```python
from build123d import *

# Parameters (mm, degrees)
F0_W     = 50.8
F0_H     = 50.8
F1_DEPTH = 50.8
F2_W     = 25.4
F2_H     = 25.4
F3_DEPTH = 25.4
F4_W     = 25.4
F4_H     = 25.4
F5_DEPTH = 25.4
F6_R     = 12.703868
F7_DEPTH = 25.4
F8_R     = 14.195008
F9_DEPTH = 25.4


with BuildPart() as f1:
    # F0 (on Front) → F1 (new body)
    with BuildSketch(Plane.XZ):
        with Locations((-25.4, 25.4)):
            Rectangle(F0_W, F0_H)
    extrude(amount=F1_DEPTH)

    # F2 (on face) → F3 (join)
    with BuildSketch(Plane.XZ.offset(50.8)):
        with Locations((-25.4, 25.4)):
            Rectangle(F2_W, F2_H)
    extrude(amount=F3_DEPTH)

    # F4 (on face) → F5 (cut)
    with BuildSketch(Plane(origin=(-50.8, 0, 0), x_dir=(0, -1, 0), z_dir=(-1, 0, 0))):
        with Locations((25.4, 25.4)):
            Rectangle(F4_W, F4_H)
    extrude(amount=-F5_DEPTH, mode=Mode.SUBTRACT)

    # F6 (on face) → F7 (cut)
    with BuildSketch(Plane.YZ):
        with Locations((-25.396969, 23.869332)):
            Circle(F6_R)
    extrude(amount=-F7_DEPTH, mode=Mode.SUBTRACT)

    # F8 (on face) → F9 (join)
    with BuildSketch(Plane(origin=(0, 0, 0), x_dir=(-1, 0, 0), z_dir=(0, 1, 0))):
        with Locations((24.574604, 25.969833)):
            Circle(F8_R)
    extrude(amount=F9_DEPTH)


solid = f1.part
```
Work out the finished part from the listing and answer in its coordinate system (mm). A direction names the side the tool comes from. Round coordinates to 2 decimals unless told otherwise and drop trailing zeros. Loops run counter-clockwise (first coordinate to the right, second up) from the corner with the lowest first, then second, coordinate; pieces in that order, holes last.
(1) Each of these flat-tipped pins is pushed along its axis until it touches: P1, Ø3.5, axis at y = -17, z = 16, coming from the -X side; P2, Ø15.5, axis at y = -27, z = 30.5, coming from the -X side; P3, Ø7.5, axis at x = -31, y = -69.5, coming from the +Z side; P4, Ø20.5, axis at x = -20.5, y = -64.5, coming from the -Z side. Where does it stop, or does it pass through?
Computed values:
P1: stops at x = -25.4
P2: stops at x = -50.8
P3: stops at z = 38.1
P4: stops at z = 12.7
(2) The part is cut by section C-C, the plane x = -36. Give the vertices of the cut face in (y, z), and give its area (3 significant figures).
Computed values:
outline: (-76.2, 12.7) - (-50.8, 12.7) - (-50.8, 0) - (0, 0) - (0, 17.55) - (25.4, 17.55) - (25.4, 34.39) - (0, 34.39) - (0, 50.8) - (-50.8, 50.8) - (-50.8, 38.1) - (-76.2, 38.1) - close; hole (-38.1, 12.7) - (-12.7, 12.7) - (-12.7, 38.1) - (-38.1, 38.1) - close
area: 3,010 mm2
(3) For faces 4 (the flat face through (-38.1, -63, 25)), 5 (the flat face through (-38, -25, 12.7)), 6 (the flat face through (-26, -63, 38.1)), 7 (the cylindrical face through (-22.727, 12.522, 40.044)), 8 (the flat face through (-12.7, -63, 25)), determine the directions among +Z, -Z, +X, -X, +Y, -Y from which every point of the face is accessible in a straight line to the end or side of a thin tool.
Computed values:
face 4: +Z, -Z, -X, -Y
face 5: -X
face 6: +Z, +X, -X, -Y
face 7: +Y
face 8: +Z, -Z, +X, -Y
(4) The part is cut by section A-A, the plane y = -24. Give the vertices of the cut face in (x, z).
Computed values:
outline: (-50.8, 0) - (0, 0) - (0, 11.24) - (-25.4, 11.24) - (-25.4, 12.7) - (-50.8, 12.7) - close; (-50.8, 38.1) - (-25.4, 38.1) - (-25.4, 36.5) - (0, 36.5) - (0, 50.8) - (-50.8, 50.8) - close
(5) Find the intervals of material crossed by L1, parallel to Z at x = -37.5, y = -13; L2, parallel to Y at x = -33, z = 34; L3, parallel to Z at x = -22, y = -29.5, in increasing order.
Computed values:
L1: z = 0 to 12.7, 38.1 to 50.8
L2: y = -76.2 to -38.1, -12.7 to 25.4
L3: z = 0 to 11.85, 35.89 to 50.8
(6) The part is cut by section D-D, the plane x = -29.5. Give the vertices of the cut face in (y, z), and give its area (3 significant figures).
Computed values:
outline: (-76.2, 12.7) - (-50.8, 12.7) - (-50.8, 0) - (0, 0) - (0, 12.66) - (25.4, 12.66) - (25.4, 39.28) - (0, 39.28) - (0, 50.8) - (-50.8, 50.8) - (-50.8, 38.1) - (-76.2, 38.1) - close; hole (-38.1, 12.7) - (-12.7, 12.7) - (-12.7, 38.1) - (-38.1, 38.1) - close
area: 3,260 mm2
(7) The part is cut by section B-B, the plane z = 18.5. Give the vertices of the cut face in (x, y), and give its area (3 significant figures).
Computed values:
outline: (-50.8, -50.8) - (-38.1, -50.8) - (-38.1, -76.2) - (-12.7, -76.2) - (-12.7, -50.8) - (0, -50.8) - (0, -36.91) - (-25.4, -36.91) - (-25.4, -38.1) - (-50.8, -38.1) - close; (-50.8, -12.7) - (-25.4, -12.7) - (-25.4, -13.88) - (0, -13.88) - (0, 0) - (-12.5, 0) - (-12.5, 25.4) - (-36.65, 25.4) - (-36.65, 0) - (-50.8, 0) - close
area: 2,610 mm2
(8) The mould has two halves that part along Z. Classify faces 1 (the flat face through (-26, -25, 0)), 2 (the flat face through (-25.4, -25, 37)), 3 (the flat face through (-26, -76.2, 26)): pulls with the +Z half, pulls with the -Z half, needs draft (parallel to the pull), parting line crosses it, or undercut.
Computed values:
face 1: pulls with the -Z half
face 2: undercut
face 3: needs draft
